Design review of the part built by this model. Coordinates are the model's own, in mm. Coordinates: 2 decimals unless noted, no trailing zeros. Order: outer loops, then holes, each group sorted by start corner. A loop starts at its lowest first (then second) coordinate and runs counter-clockwise, first axis right, second up. Notation, with made-up numbers: (9, -15.75) -> (28, -15.75) arc R30 cw to (28, 9.25) -> close; hole circle Ø7 at (-30, 59.5). An arc over 180 degrees is marked (long way). Write item = value, one per line.
```python
from build123d import *

# Parameters (mm, degrees)
SKETCH_1_R           = 1.5
SKETCH_1_R_2         = 3
EXTRUDE_1_DEPTH      = 1
SKETCH_2_W           = 46.5
SKETCH_2_H           = 120
EXTRUDE_2_DEPTH      = 1
SKETCH_7_R           = 1.5
CUT_EXTRUDE_5_DEPTH  = 10
SKETCH_8_R           = 1.5
CUT_EXTRUDE_6_DEPTH  = 10
SKETCH_10_W          = 51
SKETCH_10_H          = 30
CUT_EXTRUDE_7_DEPTH  = 10
SKETCH_11_R          = 1.5
CUT_EXTRUDE_8_DEPTH  = 65
SKETCH_12_R          = 1.5
CUT_EXTRUDE_9_DEPTH  = 10
SKETCH_13_W          = 41
SKETCH_13_H          = 30
CUT_EXTRUDE_10_DEPTH = 10
SKETCH_14_R          = 10
CUT_EXTRUDE_11_DEPTH = 10
SKETCH_16_R          = 1.5
CUT_EXTRUDE_13_DEPTH = 1
SKETCH_17_R          = 1.5
CUT_EXTRUDE_14_DEPTH = 10
SKETCH_18_W          = 92
SKETCH_18_H          = 4
CUT_EXTRUDE_15_DEPTH = 10
FILLET_2_R           = 2
SKETCH_19_R          = 10
EXTRUDE_3_DEPTH      = 1
SKETCH_20_W          = 60.5
SKETCH_20_H          = 86
CUT_EXTRUDE_16_DEPTH = 10
FILLET_3_R           = 2


with BuildPart() as part:
    # 草图1 → 凸台-拉伸1 (new body)
    with BuildSketch(Plane.XY):
        Polygon((0, 0), (-145, 0), (-112.846096908, 120), (0, 120), align=None)
        with Locations((-70, 25)):
            Circle(SKETCH_1_R, mode=Mode.SUBTRACT)
        with Locations((-90, 25)):
            Circle(SKETCH_1_R, mode=Mode.SUBTRACT)
        with Locations((-80, 15)):
            Circle(SKETCH_1_R_2, mode=Mode.SUBTRACT)
        with Locations((-70, 5)):
            Circle(SKETCH_1_R, mode=Mode.SUBTRACT)
        with Locations((-90, 5)):
            Circle(SKETCH_1_R, mode=Mode.SUBTRACT)
    extrude(amount=EXTRUDE_1_DEPTH)

    # 草图2 → 凸台-拉伸2 (add)
    with BuildSketch(Plane.XY.offset(1)):
        with Locations((23.25, 60)):
            Rectangle(SKETCH_2_W, SKETCH_2_H)
    extrude(amount=-EXTRUDE_2_DEPTH)

    # 草图7 → 切除-拉伸5 (cut)
    with BuildSketch(Plane.XY.offset(1)):
        with Locations((-102.2, 107)):
            Circle(SKETCH_7_R)
        with Locations((-90.2, 95)):
            Circle(SKETCH_7_R)
    extrude(amount=-CUT_EXTRUDE_5_DEPTH, mode=Mode.SUBTRACT)

    # 草图8 → 切除-拉伸6 (cut)
    with BuildSketch(Plane.XY.offset(1)):
        with Locations((42.5, 103)):
            Circle(SKETCH_8_R)
        with Locations((42.5, 83)):
            Circle(SKETCH_8_R)
    extrude(amount=-CUT_EXTRUDE_6_DEPTH, mode=Mode.SUBTRACT)

    # 草图10 → 切除-拉伸7 (cut)
    with BuildSketch(Plane.XY.offset(1)):
        with Locations((21, 15)):
            Rectangle(SKETCH_10_W, SKETCH_10_H)
    extrude(amount=-CUT_EXTRUDE_7_DEPTH, mode=Mode.SUBTRACT)

    # 草图11 → 切除-拉伸8 (cut)
    with BuildSketch(Plane(origin=(0, 0, 0), x_dir=(-1, 0, 0), z_dir=(0, 0, -1))):
        with Locations((76.599239768, 87.797222746)):
            Circle(SKETCH_11_R)
        with Locations((58.473084028, 79.344857511)):
            Circle(SKETCH_11_R)
        with Locations((21.314464759, 62.017508779)):
            Circle(SKETCH_11_R)
        with Locations((39.4406205, 70.469874014)):
            Circle(SKETCH_11_R)
    extrude(amount=-CUT_EXTRUDE_8_DEPTH, mode=Mode.SUBTRACT)

    # 草图12 → 切除-拉伸9 (cut)
    with BuildSketch(Plane(origin=(0, 0, 0), x_dir=(-1, 0, 0), z_dir=(0, 0, -1))):
        with Locations((81.2, 113)):
            Circle(SKETCH_12_R)
        with Locations((81.2, 93)):
            Circle(SKETCH_12_R)
    extrude(amount=-CUT_EXTRUDE_9_DEPTH, mode=Mode.SUBTRACT)

    # 草图13 → 切除-拉伸10 (cut)
    with BuildSketch(Plane(origin=(0, 0, 0), x_dir=(-1, 0, 0), z_dir=(0, 0, -1))):
        with Locations((25, 15)):
            Rectangle(SKETCH_13_W, SKETCH_13_H)
    extrude(amount=-CUT_EXTRUDE_10_DEPTH, mode=Mode.SUBTRACT)

    # 草图14 → 切除-拉伸11 (cut)
    with BuildSketch(Plane(origin=(0, 0, 0), x_dir=(-1, 0, 0), z_dir=(0, 0, -1))):
        with Locations((-28.5, 104)):
            Circle(SKETCH_14_R)
    extrude(amount=-CUT_EXTRUDE_11_DEPTH, mode=Mode.SUBTRACT)

    # 草图16 → 切除-拉伸13 (cut)
    with BuildSketch(Plane(origin=(0, 0, 0), x_dir=(-1, 0, 0), z_dir=(0, 0, -1))):
        with Locations((76.5, 115)):
            Circle(SKETCH_16_R)
        with Locations((76.5, 107)):
            Circle(SKETCH_16_R)
        with Locations((19.5, 107)):
            Circle(SKETCH_16_R)
        with Locations((19.5, 115)):
            Circle(SKETCH_16_R)
    extrude(amount=-CUT_EXTRUDE_13_DEPTH, mode=Mode.SUBTRACT)

    # 草图17 → 切除-拉伸14 (cut)
    with BuildSketch(Plane(origin=(0, 0, 0), x_dir=(-1, 0, 0), z_dir=(0, 0, -1))):
        with Locations((-14.5, 115)):
            Circle(SKETCH_17_R)
        with Locations((-34.5, 115)):
            Circle(SKETCH_17_R)
    extrude(amount=-CUT_EXTRUDE_14_DEPTH, mode=Mode.SUBTRACT)

    # 草图18 → 切除-拉伸15 (cut)
    with BuildSketch(Plane(origin=(0, 0, 0), x_dir=(-1, 0, 0), z_dir=(0, 0, -1))):
        with Locations((-0.5, 32)):
            Rectangle(SKETCH_18_W, SKETCH_18_H)
    extrude(amount=-CUT_EXTRUDE_15_DEPTH, mode=Mode.SUBTRACT)

    # 圆角2
    fillet_2_edges = [part.edges().sort_by_distance(p)[0] for p in [
        (-45.5, 0, 0.5),
        (46.5, 34, 0.5),
        (-45.5, 34, 0.5),
        (46.5, 120, 0.5),
        (-145, 0, 0.5),
        (-112.846096908, 120, 0.5),
    ]]
    fillet(fillet_2_edges, radius=FILLET_2_R)

    # 草图19 → 凸台-拉伸3 (add)
    with BuildSketch(Plane(origin=(0, 0, 0), x_dir=(-1, 0, 0), z_dir=(0, 0, -1))):
        with Locations((-28.5, 104)):
            Circle(SKETCH_19_R)
    extrude(amount=-EXTRUDE_3_DEPTH)

    # 草图20 → 切除-拉伸16 (cut)
    with BuildSketch(Plane(origin=(0, 0, 0), x_dir=(-1, 0, 0), z_dir=(0, 0, -1))):
        with Locations((-16.25, 77)):
            Rectangle(SKETCH_20_W, SKETCH_20_H)
    extrude(amount=-CUT_EXTRUDE_16_DEPTH, mode=Mode.SUBTRACT)

    # 圆角3
    fillet_3_edges = [part.edges().sort_by_distance(p)[0] for p in [
        (-14, 120, 0.5),
        (-14, 34, 0.5),
    ]]
    fillet(fillet_3_edges, radius=FILLET_3_R)


solid = part.part
```
(1) The part is to be moulded in two halves that separate along Y. For faces 1 (the cylindrical face through (-22.745, 62.468, 0.493)), 2 (the flat face through (-129, 59.71, 0.49)), 3 (the flat face through (-80, 61, 1)), say which applies: released by +Y, released by -Y, zero draft, split by the parting line, or undercut.
Report:
face_1 = undercut
face_2 = released by +Y
face_3 = zero draft
(2) We need section D-D (y = 25). Write out the cut boundary in (x, z).
Report:
outline = (-138.3, 0) -> (-91.5, 0) -> (-91.5, 1) -> (-138.3, 1) -> close; (-88.5, 0) -> (-71.5, 0) -> (-71.5, 1) -> (-88.5, 1) -> close; (-68.5, 0) -> (-45.5, 0) -> (-45.5, 1) -> (-68.5, 1) -> close
(3) Insertion check: pin 1 (1.5 mm diameter, centred on x = -62, y = 35.5, fed in from -Z); pin 2 (0.5 mm diameter, centred on y = 22.5, z = 0.5, fed in from +X). Each pin has a flat end and moves straight along its axis. Give the tip position at first contact, or say it passes through.
Report:
pin_1 = 0
pin_2 = -45.5
(4) We need section A-A (x = -81.2). Write out the cut boundary in (y, z).
Report:
outline = (0, 0) -> (12.25, 0) -> (12.25, 1) -> (0, 1) -> close; (17.75, 0) -> (91.5, 0) -> (91.5, 1) -> (17.75, 1) -> close; (94.5, 0) -> (111.5, 0) -> (111.5, 1) -> (94.5, 1) -> close; (114.5, 0) -> (120, 0) -> (120, 1) -> (114.5, 1) -> close
(5) We need section C-C (z = 0.8). Give the number of separate pieces and of enclosed holes in the cut face, and give its area (3 significant figures).
Report:
separate_pieces = 1
enclosed_holes = 17
area = 12,600 mm²
(6) We need section B-B (y = 107). Write out the cut boundary in (x, z).
Report:
outline = (-116.33, 0) -> (-103.7, 0) -> (-103.7, 1) -> (-116.33, 1) -> close; (-100.7, 0) -> (-78, 0) -> (-78, 1) -> (-100.7, 1) -> close; (-75, 0) -> (-21, 0) -> (-21, 1) -> (-75, 1) -> close; (-18, 0) -> (-14, 0) -> (-14, 1) -> (-18, 1) -> close
(7) For L1, parallel to Y at x = -19.5, z = 0.2; L2, parallel to Y at x = -70, z = 0.5; L3, parallel to X at y = 107, z = 0.3, list the stretches that pass through material, from the lowest coordinate up.
Report:
L1 = 34 to 105.5, 108.5 to 113.5, 116.5 to 120
L2 = 0 to 3.5, 6.5 to 23.5, 26.5 to 120
L3 = -116.33 to -103.7, -100.7 to -78, -75 to -21, -18 to -14
